Geometry: final body of the model. Coordinates: model frame, mm. A direction names the side the tool comes from. Coordinates: 2 decimals unless noted, no trailing zeros. Write each loop counter-clockwise with the first axis right and the second up, starting at its lowest first coordinate (ties: lowest second). Pieces come first, ordered by that corner, then holes.
Autodesk Inventor part; units mm, degrees
ref_plane "YZ Plane" through (0, 0, 0) normal (1, 0, 0) x (0, 1, 0)
ref_plane "XZ Plane" through (0, 0, 0) normal (0, 1, 0) x (-1, 0, 0)
ref_plane "XY Plane" through (0, 0, 0) normal (0, 0, 1) x (1, 0, 0)
sketch "Sketch1" plane through (0, 0, 0) normal (0, 1, 0) x (-1, 0, 0)
  line L0 (-25, 25) -> (25, 25)
  line L1 (25, 25) -> (25, -25)
  line L2 (25, -25) -> (-25, -25)
  line L3 (-25, -25) -> (-25, 25)
  line L4 (-25, 25) -> (25, -25) construction
  line L5 (25, 25) -> (-25, -25) construction
  line L6 (-30, 30) -> (30, 30) construction
  line L7 (30, 30) -> (30, -30) construction
  line L8 (30, -30) -> (-30, -30) construction
  line L9 (-30, -30) -> (-30, 30) construction
  line L10 (-30, 30) -> (30, -30) construction
  line L11 (30, 30) -> (-30, -30) construction
  line L12 (-25, 30) -> (-30, 25)
  line L13 (-30, 25) -> (-25, 30)
  line L14 (-25, 30) -> (-20, 25)
  line L15 (-20, 25) -> (-25, 20)
  line L16 (-25, 20) -> (-30, 25)
  line L17 (0, 0) -> (0, 2.49) construction
  line L18 (0, 0) -> (2.0714, 0) construction
  line L19 (25, 30) -> (30, 25)
  line L20 (25, 30) -> (20, 25)
  line L21 (20, 25) -> (25, 20)
  line L22 (25, 20) -> (30, 25)
  line L23 (-25, -30) -> (-30, -25)
  line L24 (-25, -30) -> (-20, -25)
  line L25 (-20, -25) -> (-25, -20)
  line L26 (-25, -20) -> (-30, -25)
  line L27 (25, -30) -> (20, -25)
  line L28 (25, -20) -> (30, -25)
  line L29 (25, -30) -> (30, -25)
  line L30 (20, -25) -> (25, -20)
  dimension "d0" = 50
  dimension "d1" = 50
  dimension "d2" = 60
  dimension "d3" = 60
  dimension "d4" = 5
  dimension "d5" = 5
extrude "Extrusion1" add sketch "Sketch1" along normal blind 2
fillet "Fillet1" radius 2 16 edges at (30, 1, 25) (25, 1, 30) (25, 1, 20) (25, 1, -20) (30, 1, -25) (25, 1, -30) (20, 1, -25) (-20, 1, -25) (-25, 1, -30) (-30, 1, -25) (-25, 1, -20) (-25, 1, 20) (-20, 1, 25) (-30, 1, 25) (-25, 1, 30) (20, 1, 25)
properties part number "drone"
Item 1: Pin query (flat end, axial travel): pin 1 (1 mm diameter, centred on y = 1, z = -1, fed in from -X); pin 2 (0.6 mm diameter, centred on x = -2, y = 1, fed in from +Z); pin 3 (0.6 mm diameter, centred on y = 1, z = 9, fed in from +X). Return the tip coordinate at first contact, or that it passes through.
Derived:
pin 1: stops at x = -25
pin 2: stops at z = 25
pin 3: stops at x = 25
Item 2: Section B-B, the plane z = -1. Output: boundary loops of the cut face in (x, y), plus the area to 3 significant figures.
Derived:
outline: (-25, 0) - (25, 0) - (25, 2) - (-25, 2) - close
area: 100 mm2
Item 3: Pull-direction query (Z, two-part tool) for faces 1 (the cylindrical face through (25.02, 1.01, -29.17)), 2 (the flat face through (0, 1, 25)), 3 (the flat face through (25, 1, 0)); classes: released by +Z, released by -Z, zero draft, split by the parting line, or undercut.
Derived:
face 1: released by -Z
face 2: released by +Z
face 3: undercut
Item 4: Section C-C, the plane x = -0.5. Output: boundary loops of the cut face in (y, z), plus the area to 3 significant figures.
Derived:
outline: (0, -25) - (2, -25) - (2, 25) - (0, 25) - close
area: 100 mm2
Item 5: Material intervals for probe 1 along Z at (x, y) = (17, 0.6); probe 2 along X at (y, z) = (1.75, -20), sorted ascending.
Derived:
probe 1: z = -25 to 25
probe 2: x = -25.18 to 25.18
Item 6: Set-up query: faces 4 (the flat face through (0, 1, -25)), 5 (the flat face through (-27, 1, -22)), 6 (the cylindrical face through (25.15, 1.01, 19.93)), 7 (the flat face through (22, 1, 27)). Return all of +Z, -Z, +X, -X, +Y, -Y with unobstructed straight access to the full face (end or side cutting, diameter ignored); none if empty.
Derived:
face 4: -Z, +Y, -Y
face 5: -X, +Y, -Y
face 6: +X, +Y, -Y
face 7: +Z, +Y, -Y
